Could you check a few things on this model? Use its own coordinates, in mm. Face numbers are marked on the shaded views. A direction names the side the tool comes from. Give positions to 0.01 mm unless a question says otherwise; leave off trailing zeros. Loops run counter-clockwise (first coordinate to the right, second up) from the corner with the lowest first, then second, coordinate; pieces in that order, holes last. Notation, with made-up numbers: (30.25, 86.5) - (61.25, 86.5) arc R28 cw to (61.25, 121.5) - close; hole circle Ø6 at (21, 40). An arc over 180 degrees is marked (long way). Write each question's results on one line, items separated by ' | '. Start each with the question number.
1) On a 3-axis mill with a long thin cutter (end or side, diameter ignored), from which of +Z, -Z, +X, -X, +Y, -Y can I reach the whole of each face in a straight line? I mean the marked faces 1, 2 and 3. Say none if no direction works.
2) I want a section at A-A, the plane z = 5.5. Count the separate pieces of the cut face and the enclosed holes in it, and give its area (3 significant figures).
3) If I drill on probe 1 along X at (y, z) = (-2.75, 3.75); probe 2 along X at (y, z) = (4.5, 11), over which ranges is the centre line in solid material (lowest first)? Write a range as [from, to].
4) I'm going to push flat-ended pins straight in: pin 1 (4 mm diameter, centred on x = -6.5, z = 5.5, fed in from -Y); pin 2 (2 mm diameter, centred on y = -5.5, z = 4, fed in from +X); pin 3 (2.5 mm diameter, centred on x = 9.5, z = 10.5, fed in from +Y). Where does each tip first touch, or does it pass through?
5) I want a section at B-B, the plane y = -9.25. Write out the boundary of the cut face in (x, z).
6) If we mould it in two halves opening along X, with no side actions, what happens to the marked faces 4, 5, 6 and 7? For each: +X half, -X half, draft (parallel to the pull), parting line (faces both ways), or undercut.
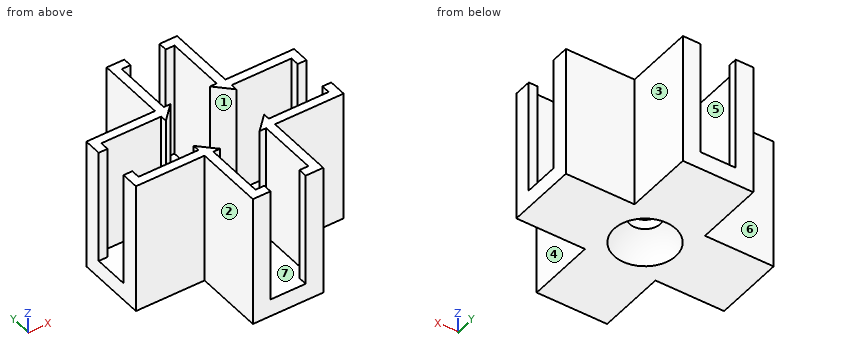
from build123d import *

# Parameters (mm, degrees)
PAD052_DEPTH          = 15
BOX006_W              = 4
BOX006_H              = 15
BOX006_DEPTH          = 12
POLARPATTERN021_COUNT = 4
PAD053_DEPTH          = 2
CYLINDER079_R         = 1.75
CYLINDER079_DEPTH     = 5


with BuildPart() as part:
    # Sketch087 → Pad052 (new body)
    with BuildSketch(Plane.XY):
        Polygon((-11.8, 4), (-4, 4), (-4, 11.8), (4, 11.8), (4, 4), (11.8, 4), (11.8, -4), (4, -4), (4, -11.8), (-4, -11.8), (-4, -4), (-11.8, -4), align=None)
        Polygon((-3, 10.8), (3, 10.8), (3, 4), (2.25, 4), (4, 2.25), (4, 3), (10.8, 3), (10.8, -3), (4, -3), (4, -2.25), (2.25, -4), (3, -4), (3, -10.8), (-3, -10.8), (-3, -4), (-2.25, -4), (-4, -2.25), (-4, -3), (-10.8, -3), (-10.8, 3), (-4, 3), (-4, 2.25), (-2.25, 4), (-3, 4), align=None, mode=Mode.SUBTRACT)
    extrude(amount=PAD052_DEPTH)

    # Box006 → Box006 (cut)
    with BuildSketch(Plane(origin=(-2, 0, 2), x_dir=(1, 0, 0), z_dir=(0, -1, 0))):
        with Locations((2, 7.5)):
            Rectangle(BOX006_W, BOX006_H)
    box006 = extrude(amount=BOX006_DEPTH, mode=Mode.SUBTRACT)

    # PolarPattern021: Box006 ×4 about axis
    polarpattern021_axis = Axis((0, 0, 0), (0, 0, 1))
    for i in range(1, POLARPATTERN021_COUNT):
        add(box006.rotate(polarpattern021_axis, i * 360 / POLARPATTERN021_COUNT), mode=Mode.SUBTRACT)

    # Sketch088 → Pad053 (join)
    with BuildSketch(Plane.XY):
        Polygon((-4, 11.8), (-4, 4), (-11.8, 4), (-11.8, -4), (-4, -4), (-4, -11.8), (4, -11.8), (4, -4), (11.8, -4), (11.8, 4), (4, 4), (4, 11.8), align=None)
    extrude(amount=PAD053_DEPTH)

    # Sphere003 → Sphere003 (revolve)
    with BuildSketch(Plane(origin=(0, 0, 0), x_dir=(-1, 0, 0), z_dir=(0, -1, 0))):
        with BuildLine():
            ThreePointArc((0, -4.5), (3.181981, -3.181981), (4.5, 0))
            Line((4.5, 0), (0, 0))
            Line((0, 0), (0, -4.5))
        make_face()
    revolve(axis=Axis((0, 0, 0), (0, 0, -1)))

    # Cylinder079 → Cylinder079 (cut)
    with BuildSketch(Plane.XY):
        Circle(CYLINDER079_R)
    extrude(amount=CYLINDER079_DEPTH, mode=Mode.SUBTRACT)

    # Sphere002 → Sphere002 (revolve, cut)
    with BuildSketch(Plane.XZ):
        with BuildLine():
            ThreePointArc((0, -3.5), (3.5, 0), (0, 3.5))
            Line((0, 3.5), (0, -3.5))
        make_face()
    revolve(axis=Axis((0, 0, 0), (0, 0, 1)), mode=Mode.SUBTRACT)


solid = part.part
Answers:
1) face 1: +Z | face 2: +Z, -Z, -X, -Y | face 3: +Z, -Z, +X, +Y
2) separate pieces: 4 | enclosed holes: 0 | area: 76.5 mm2
3) probe 1: x = [-11.8, -10.8], [-4, -3.5], [3.5, 4], [10.8, 11.8] | probe 2: x = [-4, -3], [3, 4]
4) pin 1: stops at y = -4 | pin 2: stops at x = 4 | pin 3: stops at y = 4
5) outline: (-4, 0) - (4, 0) - (4, 15) - (3, 15) - (3, 2) - (-3, 2) - (-3, 15) - (-4, 15) - close
6) face 4: +X half | face 5: undercut | face 6: draft | face 7: undercut
